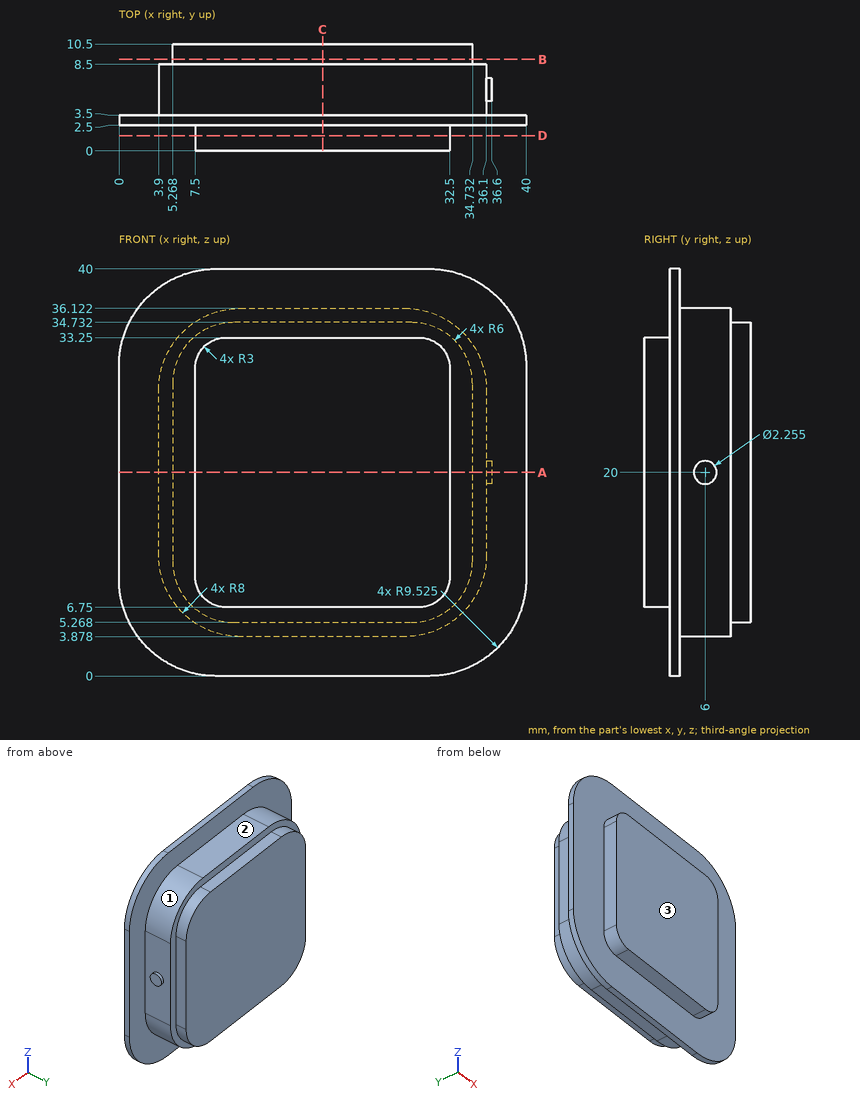
Part print with two shaded views. Sizes in mm from the minimum x, y, z corner. A direction names the side the tool comes from. Coordinates: 2 decimals unless noted, no trailing zeros. Write each loop counter-clockwise with the first axis right and the second up, starting at its lowest first coordinate (ties: lowest second). Pieces come first, ordered by that corner, then holes. Notation, with made-up numbers: (-11.5, -15) - (26.5, -15) arc R18 cw to (26.5, 19) - close; hole circle Ø4 at (-27.75, 13.25). An arc over 180 degrees is marked (long way). One line per item, written item: value. Start each with the question number.
1. Flat gauge pins, fed straight in: pin 1 (1 mm diameter, centred on x = 12, z = 22.5, fed in from -Y); pin 2 (1.6 mm diameter, centred on y = 9.5, z = 16.5, fed in from -X); pin 3 (0.6 mm diameter, centred on y = 9.5, z = 24, fed in from +X); pin 4 (1 mm diameter, centred on x = 26, y = 1, fed in from -Z). Where does each tip first touch, or does it go through?
2. Probe line 1 (Z direction, x = 26, y = 6); line 2 (X direction, y = 6.5, z = 16); line 3 (X direction, y = 0.75, z = 17.5). List the from-to ranges inside material, lowest first. Write a range as from..to.
3. Slice it at C-C (x = 20). Write the cut outline in (y, z).
4. Slice it at D-D (y = 1.5). Write the cut outline in (x, z), plus the area to 3 significant figures.
5. Tool access for the marked faces 1, 2 and 3: list every direction of +Z, -Z, +X, -X, +Y, -Y with a clear straight run to the whole face (end or side of a thin tool).
6. Slice it at B-B (y = 9). Write the cut outline in (x, z).
7. Slice it at A-A (z = 20). Write the cut outline in (x, y).
Answers below:
1. pin 1: stops at y = 0
1. pin 2: stops at x = 5.27
1. pin 3: stops at x = 34.73
1. pin 4: stops at z = 6.75
2. line 1: z = 3.88..36.12
2. line 2: x = 3.9..36.1
2. line 3: x = 7.5..32.5
3. outline: (0, 6.75) - (2.5, 6.75) - (2.5, 0) - (3.5, 0) - (3.5, 3.88) - (8.5, 3.88) - (8.5, 5.27) - (10.5, 5.27) - (10.5, 34.73) - (8.5, 34.73) - (8.5, 36.12) - (3.5, 36.12) - (3.5, 40) - (2.5, 40) - (2.5, 33.25) - (0, 33.25) - close
4. outline: (7.5, 9.75) arc R3 ccw to (10.5, 6.75) - (29.5, 6.75) arc R3 ccw to (32.5, 9.75) - (32.5, 30.25) arc R3 ccw to (29.5, 33.25) - (10.5, 33.25) arc R3 ccw to (7.5, 30.25) - close
4. area: 655 mm^2
5. face 1: +Z, +X, +Y
5. face 2: +Z, +X, -X, +Y
5. face 3: +Z, -Z, +X, -X, -Y
6. outline: (5.27, 11.27) arc R6 ccw to (11.27, 5.27) - (28.73, 5.27) arc R6 ccw to (34.73, 11.27) - (34.73, 28.73) arc R6 ccw to (28.73, 34.73) - (11.27, 34.73) arc R6 ccw to (5.27, 28.73) - close
7. outline: (0, 2.5) - (7.5, 2.5) - (7.5, 0) - (32.5, 0) - (32.5, 2.5) - (40, 2.5) - (40, 3.5) - (36.1, 3.5) - (36.1, 4.87) - (36.6, 4.87) - (36.6, 7.13) - (36.1, 7.13) - (36.1, 8.5) - (34.73, 8.5) - (34.73, 10.5) - (5.27, 10.5) - (5.27, 8.5) - (3.9, 8.5) - (3.9, 3.5) - (0, 3.5) - close
